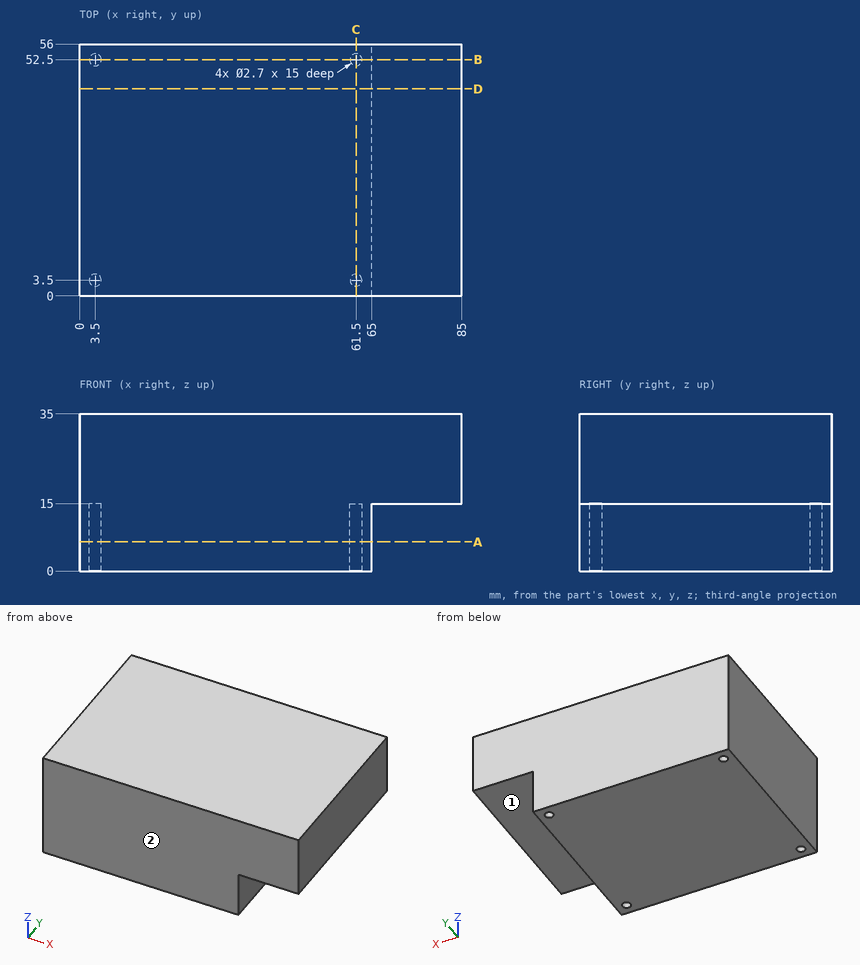
Here's the drawing with two shaded views (mm, measured from the low corner). I have some questions. A direction names the side the tool comes from. Coordinates: 2 decimals unless noted, no trailing zeros. Order: outer loops, then holes, each group sorted by start corner. A loop starts at its lowest first (then second) coordinate and runs counter-clockwise, first axis right, second up.
Q1. Which directions (+Z, -Z, +X, -X, +Y, -Y) give clear straight access to the entire face, cutting with the end or side of a thin tool? Please do the marked faces 1 and 2.
Q2. Will these pins go through, and if not, where does the flat tip stop? pin 1 (1.5 mm diameter, centred on x = 22, y = 12.5, fed in from -Z); pin 2 (2 mm diameter, centred on x = 3.5, y = 52.5, fed in from -Z); pin 3 (7.5 mm diameter, centred on y = 26.5, z = 5.5, fed in from +X).
Q3. Suppose I cut it at C-C on x = 61.5. Please give me the cut outline in (y, z), and give its area (3 significant figures).
Q4. Please list where these lines run through material, in increasing order: L1, parallel to Y at x = 61.5, z = 4.5; L2, parallel to X at y = 52.5, z = 9.75; L3, parallel to Z at x = 67, y = 19.
Q5. Suppose I cut it at B-B on y = 52.5. Please give me the cut outline in (x, z).
Q6. Suppose I cut it at A-A on z = 6.5. Please give me the cut outline in (x, y).
Q7. Suppose I cut it at D-D on y = 46. Please give me the cut outline in (x, z).
Answer:
1. face 1: -Z, +X, +Y, -Y
1. face 2: +Z, -Z, +X, -X, -Y
2. pin 1: stops at z = 0
2. pin 2: stops at z = 15
2. pin 3: stops at x = 65
3. outline: (0, 0) - (2.15, 0) - (2.15, 15) - (4.85, 15) - (4.85, 0) - (51.15, 0) - (51.15, 15) - (53.85, 15) - (53.85, 0) - (56, 0) - (56, 35) - (0, 35) - close
3. area: 1,880 mm2
4. L1: y = 0 to 2.15, 4.85 to 51.15, 53.85 to 56
4. L2: x = 0 to 2.15, 4.85 to 60.15, 62.85 to 65
4. L3: z = 15 to 35
5. outline: (0, 0) - (2.15, 0) - (2.15, 15) - (4.85, 15) - (4.85, 0) - (60.15, 0) - (60.15, 15) - (62.85, 15) - (62.85, 0) - (65, 0) - (65, 15) - (85, 15) - (85, 35) - (0, 35) - close
6. outline: (0, 0) - (65, 0) - (65, 56) - (0, 56) - close; hole circle Ø2.7 at (3.5, 3.5); hole circle Ø2.7 at (3.5, 52.5); hole circle Ø2.7 at (61.5, 3.5); hole circle Ø2.7 at (61.5, 52.5)
7. outline: (0, 0) - (65, 0) - (65, 15) - (85, 15) - (85, 35) - (0, 35) - close
